from build123d import *

# Parameters (mm, degrees)
SKETCH1_W            = 20
SKETCH1_H            = 10
BOSS_EXTRUDE1_DEPTH  = 3
M3_CLEARANCE_HOLE1_D = 3.4
FILLET3_R            = 1
CUT_EXTRUDE4_START   = -10
CUT_EXTRUDE4_DEPTH   = 10
FILLET4_R            = 0.5


# Read off the part's stored shape, not the designer's step: Cut-Extrude4
with BuildPart() as part:
    # Sketch1 → Boss-Extrude1 (new body)
    with BuildSketch(Plane(origin=(0, 0, 0), x_dir=(1, 0, 0), z_dir=(0, 1, 0))):
        with Locations((3.769230769, -2)):
            Rectangle(SKETCH1_W, SKETCH1_H)
    extrude(amount=BOSS_EXTRUDE1_DEPTH)

    # M3 Clearance Hole1 (through all)
    with Locations(Plane(origin=(0, 3, 0), x_dir=(1, 0, 0), z_dir=(0, 1, 0))):
        with Locations((-0.630769231, -2), (8.169230769, -2)):
            Hole(M3_CLEARANCE_HOLE1_D / 2)

    # Fillet3
    fillet3_edges = [part.edges().sort_by_distance(p)[0] for p in [
        (3.769230769, 3, 7),
        (13.769230769, 3, 2),
        (3.769230769, 3, -3),
        (-6.230769231, 3, 2),
    ]]
    fillet(fillet3_edges, radius=FILLET3_R)

    # Cut-Extrude4 outline → Cut-Extrude4 (cut)
    with BuildSketch(Plane.XY.offset(7).offset(CUT_EXTRUDE4_START)):
        with BuildLine():
            ThreePointArc((13.769230769, 0), (3.769230769, 0.339931125), (-6.230769231, 0))
            Line((-6.230769231, 0), (13.769230769, 0))
        make_face()
    extrude(amount=CUT_EXTRUDE4_DEPTH, mode=Mode.SUBTRACT)

    # Fillet4
    fillet4_edges = [part.edges().sort_by_distance(p)[0] for p in [
        (13.769230769, 0, 2),
        (-6.230769231, 0, 2),
    ]]
    fillet(fillet4_edges, radius=FILLET4_R)


solid = part.part
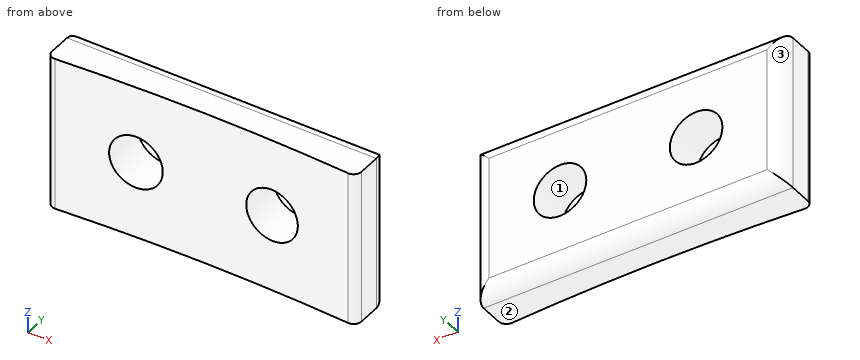
Work out the finished part from the listing and answer in its coordinate system (mm). Face numbers are marked on the shaded views. Round coordinates to 2 decimals unless told otherwise and drop trailing zeros. Write each loop counter-clockwise with the first axis right and the second up, starting at its lowest first coordinate (ties: lowest second). Pieces come first, ordered by that corner, then holes. Notation, with made-up numbers: (-15, 65) -> (-4, 65) arc R24 cw to (-4, 89) -> close; hole circle Ø5 at (54.25, -13). An arc over 180 degrees is marked (long way). Answer as CSV lines item,"result". Start each with the question number.
(1) The mould has two halves that part along Z. Classify the marked faces 1, 2 and 3: +Z half, -Z half, draft (parallel to the pull), parting line (faces both ways), or undercut.
(2) The part is cut by section B-B, the plane y = 1.35. Give the vertices of the cut face in (x, z), then the cut area to 3 significant figures.
(3) The part is cut by section A-A, the plane z = 3.5. Give the vertices of the cut face in (x, y), then the cut area to 3 significant figures.
(4) The part is cut by section D-D, the plane x = 2. Give the vertices of the cut face in (y, z).
(5) Each of these flat-tipped pins is pushed along its axis until it touches: pin 1 (1.5 mm diameter, centred on x = -4, z = 5.5, fed in from -Y); pin 2 (2 mm diameter, centred on x = -0.63, z = 2, fed in from -Y). Where does it stop, or does it pass through?
(6) Find the intervals of material crossed by probe 1 along X at (y, z) = (2.3, 3); probe 2 along Y at (x, z) = (-2.25, 4.5); probe 3 along Z at (x, y) = (-1.5, 1), in increasing order.
(7) The part is cut by section C-C, the plane z = -0.5. Give the vertices of the cut face in (x, y).
Output values:
1,face 1,"undercut"
1,face 2,"-Z half"
1,face 3,"draft"
2,outline,"(-6.23, -3) -> (13.77, -3) -> (13.77, 7) -> (-6.23, 7) -> close; hole circle Ø3.4 at (-0.63, 2); hole circle Ø3.4 at (8.17, 2)"
2,area,"182 mm²"
3,outline,"(-6.23, 0.53) arc R0.5 ccw to (-5.7, 0.04) arc R147.26 cw to (-1.43, 0.25) -> (-1.43, 3) -> (-5.23, 3) arc R1 ccw to (-6.23, 2) -> close; (0.17, 0.3) arc R147.26 cw to (7.37, 0.3) -> (7.37, 3) -> (0.17, 3) -> close; (8.97, 0.25) arc R147.26 cw to (13.24, 0.04) arc R0.5 ccw to (13.77, 0.53) -> (13.77, 2) arc R1 ccw to (12.77, 3) -> (8.97, 3) -> close"
3,area,"46.2 mm²"
4,outline,"(0.33, -3) -> (2, -3) arc R1 ccw to (3, -2) -> (3, 6) arc R1 ccw to (2, 7) -> (0.33, 7) -> close"
5,pin 1,"stops at y = 0.09"
5,pin 2,"passes through"
6,probe 1,"x = -6.18 to -2.01, 0.74 to 6.79, 9.54 to 13.72"
6,probe 2,"y = 0.22 to 3"
6,probe 3,"z = -3 to 0.54, 3.46 to 7"
7,outline,"(-6.23, 0.53) arc R0.5 ccw to (-5.7, 0.04) arc R147.26 cw to (13.24, 0.04) arc R0.5 ccw to (13.77, 0.53) -> (13.77, 2) arc R1 ccw to (12.77, 3) -> (-5.23, 3) arc R1 ccw to (-6.23, 2) -> close"
